Can you work these out from the model? Positions are in its coordinate system, mm. Face numbers are marked on the shaded views. A direction names the side the tool comes from. Round coordinates to 2 decimals unless told otherwise and drop trailing zeros. Loops run counter-clockwise (first coordinate to the right, second up) from the corner with the lowest first, then second, coordinate; pieces in that order, holes last. Notation, with made-up numbers: (74, 22.25) -> (128, 22.25) arc R22 cw to (128, 39.25) -> close; hole circle Ø11 at (-6.75, 86.25). An arc over 180 degrees is marked (long way). Answer as a JSON object with one key per item and string values.
Autodesk Inventor part; units mm, degrees
ref_plane "YZ Plane" through (0, 0, 0) normal (1, 0, 0) x (0, 1, 0)
ref_plane "XZ Plane" through (0, 0, 0) normal (0, 1, 0) x (-1, 0, 0)
ref_plane "XY Plane" through (0, 0, 0) normal (0, 0, 1) x (1, 0, 0)
sketch "Sketch1" plane through (0, 0, 0) normal (0, 0, 1) x (1, 0, 0)
  circle A0 centre (0, 0) radius 11
  circle A1 centre (0, 0) radius 4
  dimension "d0" = 22
  dimension "d3" = 8
extrude "Extrusion2" add sketch "Sketch1" along normal mid plane 4
sketch "Sketch2" plane through (0, 0, 2) normal (0, 0, 1) x (1, 0, 0)
  circle A0 centre (0, 0) radius 4
  circle A1 centre (0, 0) radius 11
  circle A2 centre (0, 0) radius 5
  circle A3 centre (0, 0) radius 4
  dimension "d6" = 10
  dimension "d7" = 8
extrude "Extrusion3" add sketch "Sketch2" along normal blind 1 contours A2
sketch "Sketch3" plane through (0, 0, 2) normal (0, 0, 1) x (1, 0, 0)
  circle A0 centre (0, 0) radius 5
  circle A1 centre (0, -8) radius 0.8657
  circle A2 centre (8, 0) radius 0.9464
  circle A3 centre (0, 8) radius 0.9341
  circle A4 centre (-8, 0) radius 0.9592
  dimension "d10" = 8
  dimension "d11" = 8
  dimension "d12" = 8
  dimension "d13" = 8
extrude "Extrusion4" cut sketch "Sketch3" against normal up to surface (4 mm away) contours A1 | A2 | A3 | A4
sketch "Sketch4" plane through (0, 0, -2) normal (0, 0, -1) x (-1, 0, 0)
  circle A0 centre (0, 0) radius 4
  circle A1 centre (0, 0) radius 11
  circle A2 centre (0, 0) radius 4
  circle A3 centre (0, 0) radius 5
  dimension "d16" = 10
extrude "Extrusion5" add sketch "Sketch4" along normal blind 10 contours A3
fillet "Fillet1" radius 0.25 4 edges at (-11, 0, -2) (-11, 0, 2) (5, 0, -12) (-5, 0, 3)
properties part number "Z Akse gevindstang møtrik" material "Brass, Soft Yellow"
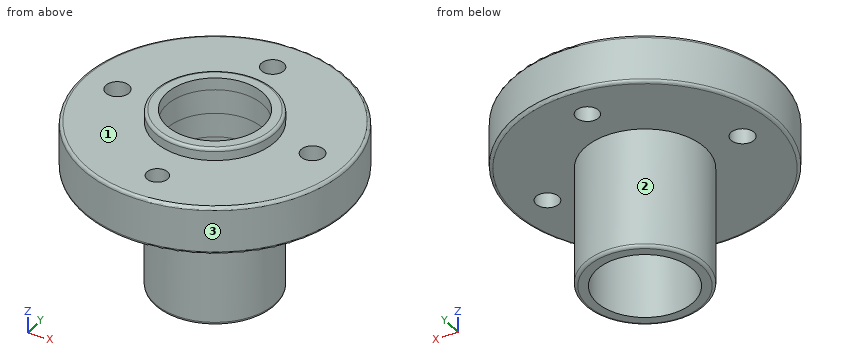
Q1. If I drill on L1, parallel to Y at x = 0, z = 0.2; L2, parallel to Y at x = 0, z = -7.25; L3, parallel to Z at x = 2, y = 9, over which ranges is the centre line in solid material (lowest first)? Write a range as [from, to].
Determined:
{"L1": "[-11, -8.87], [-7.13, -4], [4, 7.07], [8.93, 11]", "L2": "[-5, -4], [4, 5]", "L3": "[-2, 2]"}
Q2. I'm going to push flat-ended pins straight in: pin 1 (1.5 mm diameter, centred on x = 0, y = 8, fed in from +Z); pin 2 (2.5 mm diameter, centred on x = 8, y = 0, fed in from +Z); pin 3 (1 mm diameter, centred on x = -3, y = 7, fed in from -Z); pin 4 (1 mm diameter, centred on y = -4.5, z = -1, fed in from -X). Where does each tip first touch, or does it pass through?
Determined:
{"pin 1": "through", "pin 2": "z = 2", "pin 3": "z = -2", "pin 4": "x = -10.25"}
Q3. On a 3-axis mill with a long thin cutter (end or side, diameter ignored), from which of +Z, -Z, +X, -X, +Y, -Y can I reach the whole of each face in a straight line? I mean the marked faces 1, 2 and 3. Say none if no direction works.
Determined:
{"face 1": "+Z", "face 2": "-Z", "face 3": "+Z, -Z"}
Q4. I want a section at B-B, the plane z = 1.25. Write out the boundary of the cut face in (x, y), then the cut area to 3 significant figures.
Determined:
{"outline": "circle Ø22 at (0, 0); hole circle Ø1.92 at (-8, 0); hole circle Ø8 at (0, 0); hole circle Ø1.87 at (0, 8); hole circle Ø1.73 at (0, -8); hole circle Ø1.89 at (8, 0)", "area": "319 mm²"}
Q5. I want a section at C-C, the plane z = -7.75. Write out the boundary of the cut face in (x, y).
Determined:
{"outline": "circle Ø10 at (0, 0); hole circle Ø8 at (0, 0)"}
Q6. I want a section at A-A, the plane y = 0. Give the number of separate pieces and of enclosed holes in the cut face, then the cut area to 3 significant figures.
Determined:
{"separate pieces": "4", "enclosed holes": "0", "area": "62.6 mm²"}
